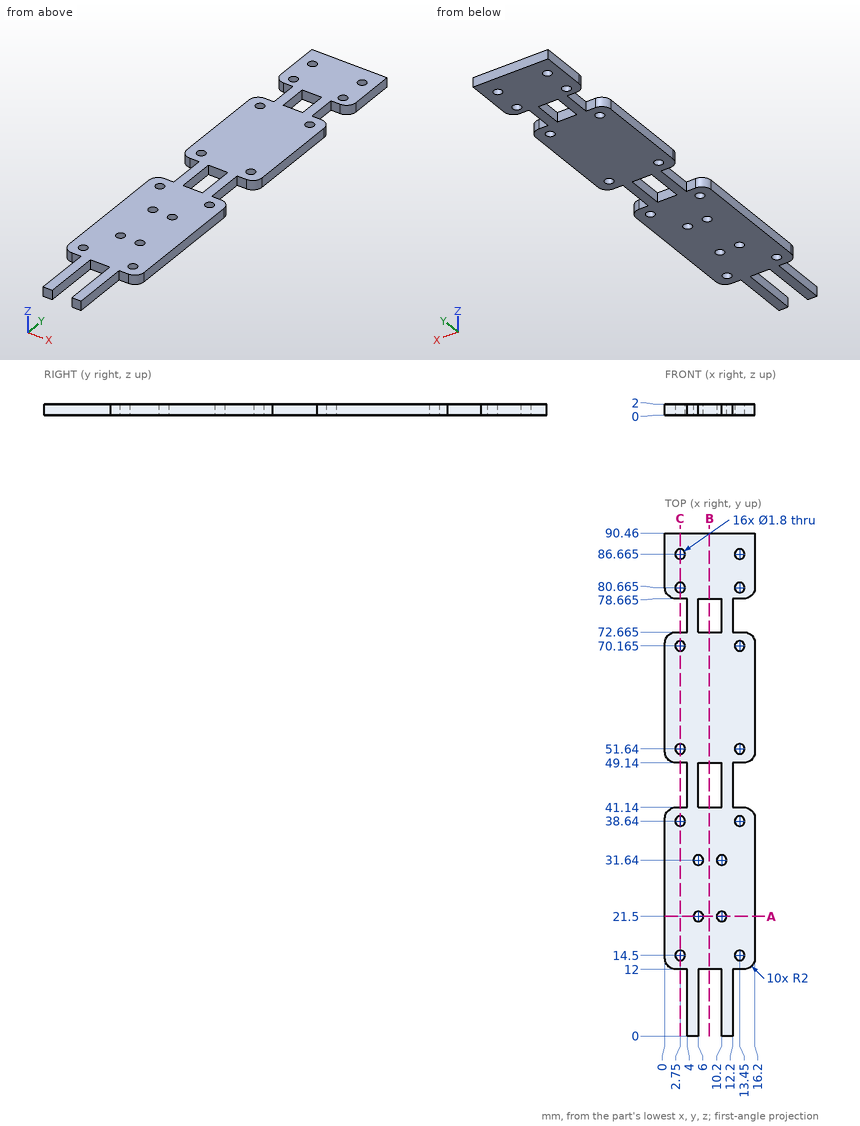
Here's the drawing with two shaded views (mm, measured from the low corner). I have some questions. Coordinates: 2 decimals unless noted, no trailing zeros. Write each loop counter-clockwise with the first axis right and the second up, starting at its lowest first coordinate (ties: lowest second). Pieces come first, ordered by that corner, then holes. Notation, with made-up numbers: M 80,10 L 98,10 A24 cw 98,25 Z; hole C -40,40.25 d1. An arc over 180 degrees is marked long. Use one line per item in the form item = value.
Q1. For P1, Ø1, axis at y = 46, z = 1.5, coming from the -X side, with a flat end and sliding along its axis, tell me the tip position at first contact or that it passes through.
Model answer:
P1 = 4
Q2. I need wall thicknesses on line 1 along X through (y, z) = (38.64, 1.1); line 2 along Y through (x, z) = (7.75, 1.2) (3 decimals); line 3 along X through (y, z) = (76.5, 1.7). Which ranges of each line are inside material? Lowest first, please. Write a range as from..to.
Model answer:
line_1 = 0..1.85, 3.65..12.55, 14.35..16.2
line_2 = 12..41.14, 49.14..72.665, 78.665..90.46
line_3 = 4..6, 10.2..12.2
Q3. If we section it at A-A (y = 21.5): Write out the boundary of the cut face in (x, z).
Model answer:
outline = M 0,0 L 5.1,0 L 5.1,2 L 0,2 Z; M 6.9,0 L 9.3,0 L 9.3,2 L 6.9,2 Z; M 11.1,0 L 16.2,0 L 16.2,2 L 11.1,2 Z
Q4. If we section it at B-B (x = 8): Write out the boundary of the cut face in (y, z) (3 decimals), then the cut area to 3 significant figures.
Model answer:
outline = M 12,0 L 41.14,0 L 41.14,2 L 12,2 Z; M 49.14,0 L 72.665,0 L 72.665,2 L 49.14,2 Z; M 78.665,0 L 90.46,0 L 90.46,2 L 78.665,2 Z
area = 129 mm^2
Q5. If we section it at C-C (x = 2.75): State how many separate pieces and enclosed holes the cut face has, then the cut area to 3 significant figures.
Model answer:
separate_pieces = 9
enclosed_holes = 0
area = 107 mm^2
